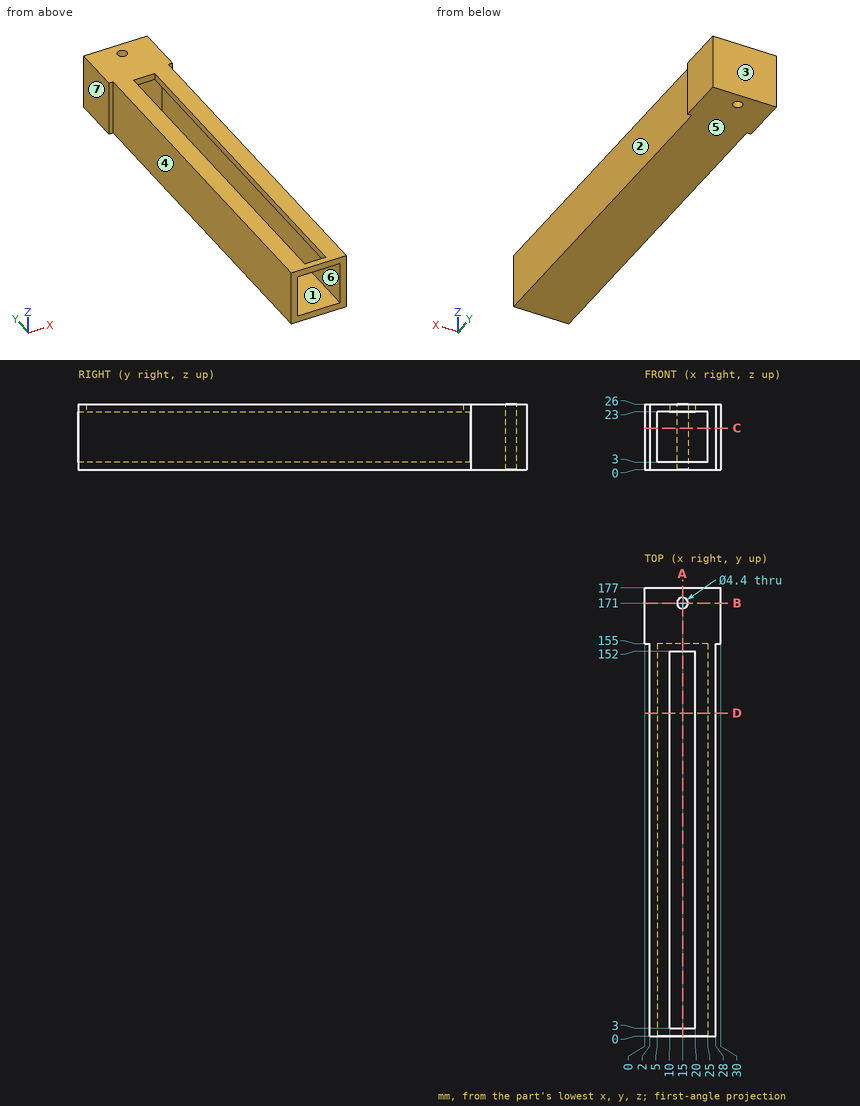
Verification items for this drawing (mm, ordinates from the low corner). A direction names the side the tool comes from. Give positions to 0.01 mm unless a question says otherwise; leave off trailing zeros. Loops run counter-clockwise (first coordinate to the right, second up) from the corner with the lowest first, then second, coordinate; pieces in that order, holes last. Notation, with made-up numbers: M -37.75,31.25 L -2.75,31.25 A22 cw -2.75,49.25 Z; hole C 89,-6 d10. An arc over 180 degrees is marked long. Write item = value, one per line. Start each with the question number.
1. Draft check along X on the marked faces 5, 6 and 7. Enter one of: +X half, -X half, draft (parallel to the pull), parting line (faces both ways), or undercut.
2. Go/stop test with flat-tipped pins: P1, Ø0.9, axis at y = 83, z = 24.5, coming from the +X side; P2, Ø6, axis at x = 18.5, z = 15.5, coming from the -Y side; P3, Ø13, axis at y = 85, z = 15, coming from the -X side. Record where each tip stops, or that it passes through.
3. Thickness scan on probe 1 along Y at (x, z) = (15, 14.75); probe 2 along Z at (x, y) = (22.5, 46); probe 3 along X at (y, z) = (97, 21). Record the ranges inside material, lowest first.
4. Section check A-A, the plane x = 15. Enter the section's corners in (y, z), plus the area to 3 significant figures.
5. Tool access check on the marked faces 1, 2, 3 and 4. Record the directions out of +Z, -Z, +X, -X, +Y, -Y that give a thin tool (end or side, any length) a straight path to the whole face; none if there is none.
6. Section check C-C, the plane z = 16.5. Enter the section's corners in (x, y).
7. Section check B-B, the plane y = 171. Enter the section's corners in (x, z).
8. Section check D-D, the plane y = 127.5. Enter the section's corners in (x, z), plus the area to 3 significant figures.
Values follow:
q1.face_5 = draft
q1.face_6 = undercut
q1.face_7 = -X half
q2.P1 = 28
q2.P2 = 155
q2.P3 = 2
q3.probe_1 = 155 to 168.8, 173.2 to 177
q3.probe_2 = 0 to 3, 23 to 26
q3.probe_3 = 2 to 5, 25 to 28
q4.outline = M 0,0 L 168.8,0 L 168.8,26 L 152,26 L 152,23 L 155,23 L 155,3 L 0,3 Z; M 0,23 L 3,23 L 3,26 L 0,26 Z; M 173.2,0 L 177,0 L 177,26 L 173.2,26 Z
q4.area = 941 mm^2
q5.face_1 = -Y
q5.face_2 = +Z, -Z, +X, -Y
q5.face_3 = +Z, -Z, +X, -X, +Y
q5.face_4 = +Z, -Z, -X, -Y
q6.outline = M 0,155 L 2,155 L 2,0 L 5,0 L 5,155 L 25,155 L 25,0 L 28,0 L 28,155 L 30,155 L 30,177 L 0,177 Z; hole C 15,171 d4.4
q7.outline = M 0,0 L 12.8,0 L 12.8,26 L 0,26 Z; M 17.2,0 L 30,0 L 30,26 L 17.2,26 Z
q8.outline = M 2,0 L 28,0 L 28,26 L 20,26 L 20,23 L 25,23 L 25,3 L 5,3 L 5,23 L 10,23 L 10,26 L 2,26 Z
q8.area = 246 mm^2
